Could you check a few things on this model? Use its own coordinates, in mm. Coordinates: 2 decimals unless noted, no trailing zeros. Order: outer loops, then holes, each group sorted by start corner. A loop starts at its lowest first (then second) coordinate and runs counter-clockwise, first axis right, second up. Notation, with made-up numbers: M -37.5,-19.5 L 15.5,-19.5 A25 cw 15.5,13.5 Z; hole C -20,30 d3. An arc over 180 degrees is marked long. Put each result on its own line as item: value. Start each with the question number.
```python
from build123d import *

# Parameters (mm, degrees)
F0_W     = 51
F0_H     = 7
F1_DEPTH = 3.75
F2_R     = 2
F3_R     = 2
F4_R     = 2
F5_R     = 2
F6_R     = 1.5
F7_DEPTH = 3.5
F8_R     = 1.5
F9_DEPTH = 3.5


with BuildPart() as f1:
    # F0 (on Top) → F1 (new body, symmetric)
    with BuildSketch(Plane.XY):
        Rectangle(F0_W, F0_H)
    extrude(amount=F1_DEPTH, both=True)

    # F2
    f2_edges = [f1.edges().sort_by_distance(p)[0] for p in [
        (-25.5, 0, 3.75),
    ]]
    fillet(f2_edges, radius=F2_R)

    # F3
    f3_edges = [f1.edges().sort_by_distance(p)[0] for p in [
        (-25.5, 0, -3.75),
    ]]
    fillet(f3_edges, radius=F3_R)

    # F4
    f4_edges = [f1.edges().sort_by_distance(p)[0] for p in [
        (25.5, 0, 3.75),
    ]]
    fillet(f4_edges, radius=F4_R)

    # F5
    f5_edges = [f1.edges().sort_by_distance(p)[0] for p in [
        (25.5, 0, -3.75),
    ]]
    fillet(f5_edges, radius=F5_R)

    # F6 (on Front) → F7 (intersect, symmetric)
    with BuildSketch(Plane.XZ):
        with BuildLine():
            ThreePointArc((-25.5, -1.75), (-24.9142135624, -3.1642135624), (-23.5, -3.75))
            Line((-23.5, -3.75), (23.5, -3.75))
            ThreePointArc((23.5, -3.75), (24.9142135624, -3.1642135624), (25.5, -1.75))
            Line((25.5, -1.75), (25.5, 1.75))
            ThreePointArc((25.5, 1.75), (24.9142135624, 3.1642135624), (23.5, 3.75))
            Line((23.5, 3.75), (-23.5, 3.75))
            ThreePointArc((-23.5, 3.75), (-24.9142135624, 3.1642135624), (-25.5, 1.75))
            Line((-25.5, 1.75), (-25.5, -1.75))
        make_face()
        with Locations((-21.5, 0)):
            Circle(F6_R, mode=Mode.SUBTRACT)
        with Locations((21.5, 0)):
            Circle(F6_R, mode=Mode.SUBTRACT)
    extrude(amount=F7_DEPTH, both=True, mode=Mode.INTERSECT)

    # F8 (on Front) → F9 (cut, symmetric)
    with BuildSketch(Plane.XZ):
        with Locations((-15.1026989078, 0)):
            Circle(F8_R)
        with Locations((12.8973010922, 0)):
            Circle(F8_R)
    extrude(amount=F9_DEPTH, both=True, mode=Mode.SUBTRACT)


solid = f1.part
```
Item 1: If we section it at B-B on y = -1.75: Write out the boundary of the cut face in (x, z), then the cut area to 3 significant figures.
Item 2: If we section it at D-D on x = 12.5: Write out the boundary of the cut face in (y, z).
Item 3: If we mould it in two halves opening along Z, with no side actions, what happens to faces 1 (the cylindrical face through (20, 0, 0)), 2 (the flat face through (-25.5, 0, 0)), 3 (the flat face through (0, 0, -3.75)), 4 (the cylindrical face through (-23, 0, 0))? For each: released by +Z, released by -Z, zero draft, split by the parting line, or undercut.
Item 4: I need wall thicknesses on probe 1 along Z at (x, y) = (21.5, -1.5); probe 2 along X at (y, z) = (-0.75, -0.25); probe 3 along X at (y, z) = (-1.25, 2.75). Which ranges of each line are inside material? Lowest first, please.
Item 5: If we section it at A-A on z = 0: Write out the boundary of the cut face in (x, y), then the cut area to 3 significant figures.
Item 6: If we section it at C-C on x = 21.5: Write out the boundary of the cut face in (y, z).
Geometry check:
1. outline: M -25.5,-1.75 A2 ccw -23.5,-3.75 L 23.5,-3.75 A2 ccw 25.5,-1.75 L 25.5,1.75 A2 ccw 23.5,3.75 L -23.5,3.75 A2 ccw -25.5,1.75 Z; hole C -21.5,0 d3; hole C -15.1,0 d3; hole C 12.9,0 d3; hole C 21.5,0 d3
1. area: 351 mm²
2. outline: M -3.5,-3.75 L 3.5,-3.75 L 3.5,-1.45 L -3.5,-1.45 Z; M -3.5,1.45 L 3.5,1.45 L 3.5,3.75 L -3.5,3.75 Z
3. face 1: undercut
3. face 2: zero draft
3. face 3: released by -Z
3. face 4: undercut
4. probe 1: z = -3.75 to -1.5, 1.5 to 3.75
4. probe 2: x = -25.5 to -22.98, -20.02 to -16.58, -13.62 to 11.42, 14.38 to 20.02, 22.98 to 25.5
4. probe 3: x = -25.23 to 25.23
5. outline: M -25.5,-3.5 L -23,-3.5 L -23,3.5 L -25.5,3.5 Z; M -20,-3.5 L -16.6,-3.5 L -16.6,3.5 L -20,3.5 Z; M -13.6,-3.5 L 11.4,-3.5 L 11.4,3.5 L -13.6,3.5 Z; M 14.4,-3.5 L 20,-3.5 L 20,3.5 L 14.4,3.5 Z; M 23,-3.5 L 25.5,-3.5 L 25.5,3.5 L 23,3.5 Z
5. area: 273 mm²
6. outline: M -3.5,-3.75 L 3.5,-3.75 L 3.5,-1.5 L -3.5,-1.5 Z; M -3.5,1.5 L 3.5,1.5 L 3.5,3.75 L -3.5,3.75 Z
